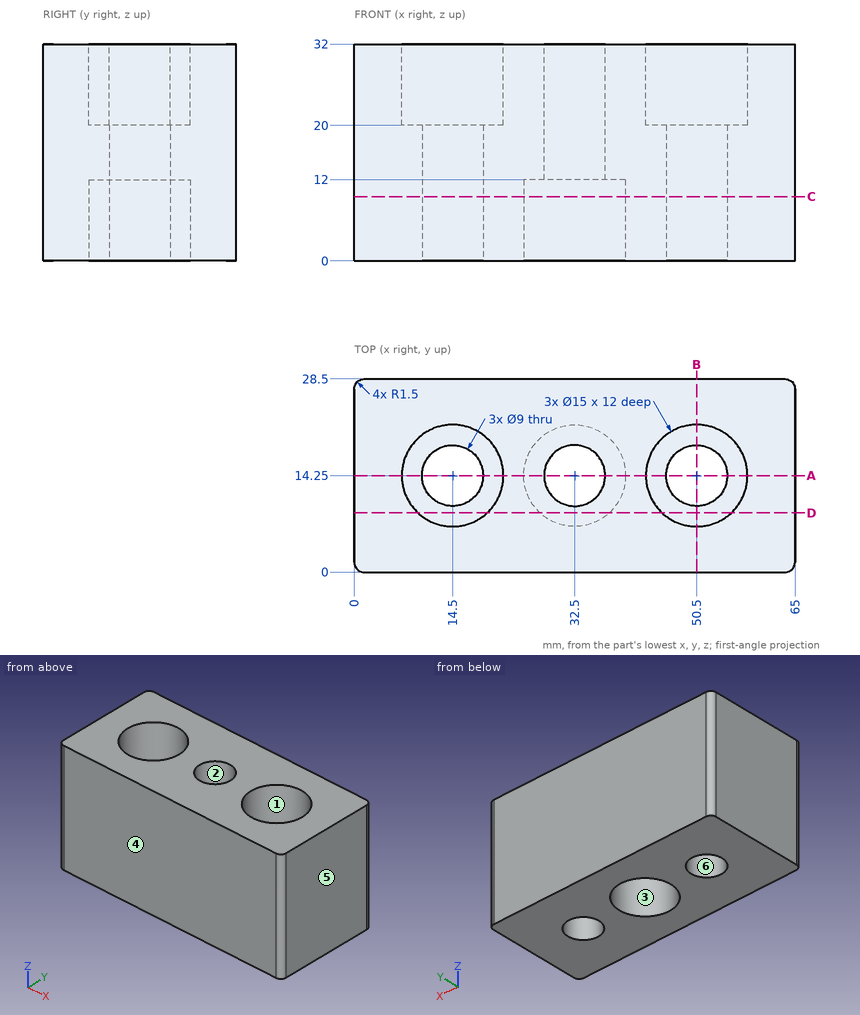
Geometry check sheet. Reference: drawing and pictorial views, mm from the part's lowest x, y, z. A direction names the side the tool comes from. Coordinates: 2 decimals unless noted, no trailing zeros. Loops run counter-clockwise (first coordinate to the right, second up) from the corner with the lowest first, then second, coordinate; pieces in that order, holes last. Notation, with made-up numbers: (-0.5, 0.5) -> (42.5, 0.5) arc R14 cw to (42.5, 27.5) -> close; hole circle Ø8 at (59, 61.25). An arc over 180 degrees is marked (long way). Put each result on its own line as item: value.
1) Cross-section at D-D on y = 8.75. Record the boundary of the cut face in (x, z), plus the area to 3 significant figures.
Result set:
outline: (0, 0) -> (27.4, 0) -> (27.4, 12) -> (37.6, 12) -> (37.6, 0) -> (65, 0) -> (65, 32) -> (55.6, 32) -> (55.6, 20) -> (45.4, 20) -> (45.4, 32) -> (19.6, 32) -> (19.6, 20) -> (9.4, 20) -> (9.4, 32) -> (0, 32) -> close
area: 1,710 mm^2
2) Thickness scan on line 1 (X direction, y = 20.25, z = 26); line 2 (Y direction, x = 50.5, z = 9.75); line 3 (X direction, y = 15.25, z = 15.5). Record the ranges inside material, lowest first.
Result set:
line 1: x = 0 to 10, 19 to 46, 55 to 65
line 2: y = 0 to 9.75, 18.75 to 28.5
line 3: x = 0 to 10.11, 18.89 to 28.11, 36.89 to 46.11, 54.89 to 65
3) Cross-section at B-B on x = 50.5. Record the boundary of the cut face in (y, z), plus the area to 3 significant figures.
Result set:
outline: (0, 0) -> (9.75, 0) -> (9.75, 20) -> (6.75, 20) -> (6.75, 32) -> (0, 32) -> close; (18.75, 0) -> (28.5, 0) -> (28.5, 32) -> (21.75, 32) -> (21.75, 20) -> (18.75, 20) -> close
area: 552 mm^2
4) Release check for a two-part mould opening along X. For the marked faces 4, 5 and 6 record: released by +X, released by -X, zero draft, split by the parting line, or undercut.
Result set:
face 4: zero draft
face 5: released by +X
face 6: undercut
5) Cross-section at C-C on z = 9.5. Record the boundary of the cut face in (x, y), plus the area to 3 significant figures.
Result set:
outline: (0, 1.5) arc R1.5 ccw to (1.5, 0) -> (63.5, 0) arc R1.5 ccw to (65, 1.5) -> (65, 27) arc R1.5 ccw to (63.5, 28.5) -> (1.5, 28.5) arc R1.5 ccw to (0, 27) -> close; hole circle Ø9 at (14.5, 14.25); hole circle Ø15 at (32.5, 14.25); hole circle Ø9 at (50.5, 14.25)
area: 1,550 mm^2
6) Tool access check on the marked faces 1, 2 and 3. Record the directions out of +Z, -Z, +X, -X, +Y, -Y that give a thin tool (end or side, any length) a straight path to the whole face; none if there is none.
Result set:
face 1: +Z
face 2: +Z, -Z
face 3: -Z
7) Cross-section at A-A on y = 14.25. Record the boundary of the cut face in (x, z).
Result set:
outline: (0, 0) -> (10, 0) -> (10, 20) -> (7, 20) -> (7, 32) -> (0, 32) -> close; (19, 0) -> (25, 0) -> (25, 12) -> (28, 12) -> (28, 32) -> (22, 32) -> (22, 20) -> (19, 20) -> close; (37, 12) -> (40, 12) -> (40, 0) -> (46, 0) -> (46, 20) -> (43, 20) -> (43, 32) -> (37, 32) -> close; (55, 0) -> (65, 0) -> (65, 32) -> (58, 32) -> (58, 20) -> (55, 20) -> close
